The drawing under review shows one solid part. Ordinate dimensions are in mm from its lowest x, y, z. A direction names the side the tool comes from. Give positions to 0.01 mm unless a question says otherwise; leave off trailing zeros. Write each loop counter-clockwise with the first axis right and the second up, starting at its lowest first coordinate (ties: lowest second). Pieces come first, ordered by that corner, then holes. Notation, with made-up numbers: (-20, 84.25) -> (-3, 84.25) arc R22 cw to (-3, 123.25) -> close; hole circle Ø11 at (-38.75, 84.5). An arc over 180 degrees is marked (long way). Answer as a JSON object with one key per item and string values.
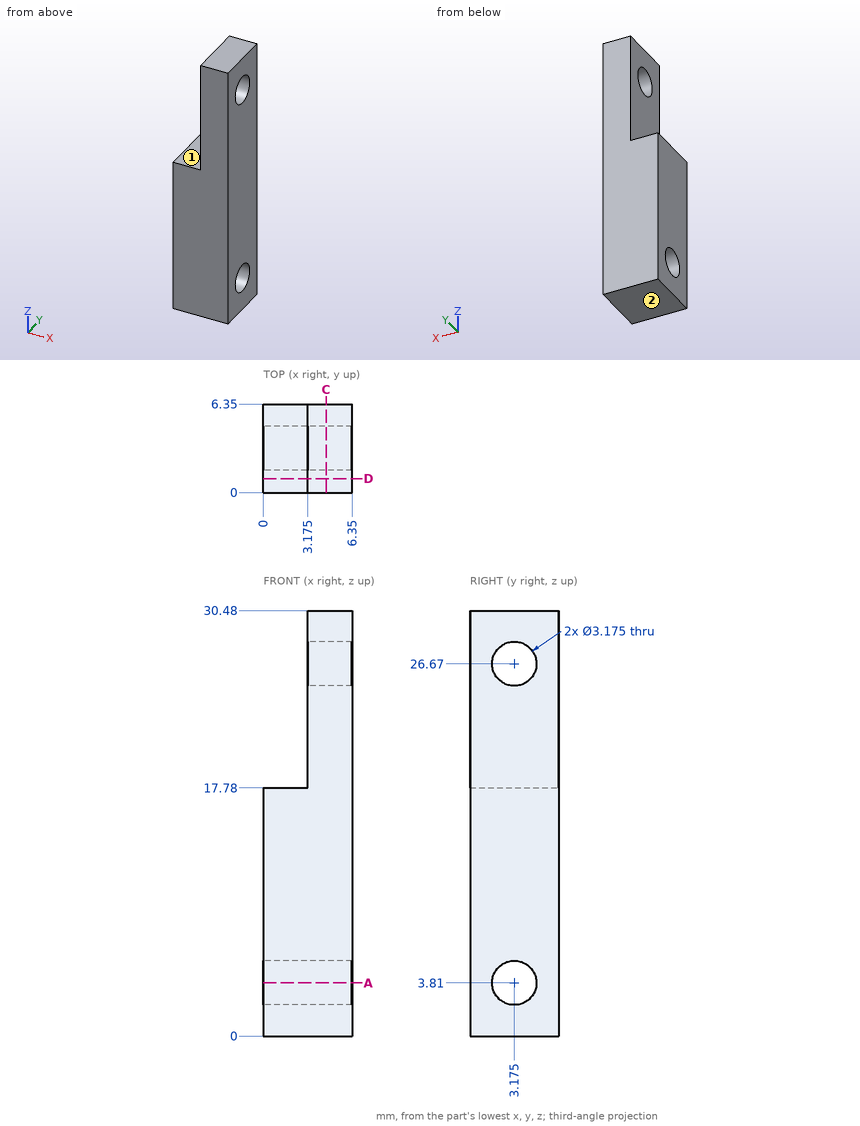
(1) For line 1 along Y through (x, z) = (4.25, 3.81); line 2 along Z through (x, y) = (4, 4.5); line 3 along Z through (x, y) = (4.5, 3), list the stretches that pass through material, from the lowest coordinate up.
Here are the results:
{"line 1": "y = 0 to 1.59, 4.76 to 6.35", "line 2": "z = 0 to 2.94, 4.68 to 25.8, 27.54 to 30.48", "line 3": "z = 0 to 2.23, 5.39 to 25.09, 28.25 to 30.48"}
(2) We need section C-C, the plane x = 4.5. Give the number of separate pieces and of enclosed holes in the cut face, then the cut area to 3 significant figures.
Here are the results:
{"separate pieces": "1", "enclosed holes": "2", "area": "178 mm²"}
(3) We need section D-D, the plane y = 1. State the section outline as (x, z) points (3 decimals), then the cut area to 3 significant figures.
Here are the results:
{"outline": "(0, 0) -> (6.35, 0) -> (6.35, 30.48) -> (3.175, 30.48) -> (3.175, 17.78) -> (0, 17.78) -> close", "area": "153 mm²"}
(4) Clearance check with a flat-ended pin moving along its axis: pin 1 (1.9 mm diameter, centred on y = 3, z = 22.5, fed in from -X) (3 decimals). State where the tip first meets the part, or that it passes through.
Here are the results:
{"pin 1": "stops at x = 3.175"}
(5) For the marked faces 1 and 2, list the 3-axis set-ups (+Z, -Z, +X, -X, +Y, -Y) from which the entire face can be reached by the end or side of a thin tool; tool diameter is ignored.
Here are the results:
{"face 1": "+Z, -X, +Y, -Y", "face 2": "-Z, +X, -X, +Y, -Y"}
(6) We need section A-A, the plane z = 3.81. State the section outline as (x, y) points.
Here are the results:
{"outline": "(0, 0) -> (6.35, 0) -> (6.35, 1.59) -> (0, 1.59) -> close; (0, 4.76) -> (6.35, 4.76) -> (6.35, 6.35) -> (0, 6.35) -> close"}
